Can you work these out from the drawing? Everything is in mm from the part's minimum corner. Coordinates: 2 decimals unless noted, no trailing zeros. Order: outer loops, then holes, each group sorted by start corner. A loop starts at its lowest first (then second) coordinate and runs counter-clockwise, first axis right, second up. Notation, with made-up numbers: (86.25, 73) - (90.25, 73) arc R22 cw to (90.25, 92) - close; hole circle Ø8 at (42, 71.25). An arc over 180 degrees is marked (long way). Use a Markdown table: item, result. Add a question column.
(1) I want a section at B-B (z = 1.2). List the corners of the cut face in (x, y) for me, and give its area (3 significant figures).
(2) We'd pull the mould along Y, two halves only. Please class the marked faces 1, 2 and 3: pulls with the +Y half, pulls with the -Y half, needs draft (parallel to the pull), parting line crosses it, or undercut.
(3) I want a section at C-C (y = 3). List the corners of the cut face in (x, z) for me.
(4) If I drill on L1, parallel to Z at x = 1.35, y = 5.25; L2, parallel to Z at x = 0.4, y = 4; L3, parallel to X at y = 9.5, z = 1.05, over which ranges is the centre line in solid material (lowest first)? Write a range as [from, to].
(5) I want a section at A-A (x = 1.4). List the corners of the cut face in (y, z) for me, and give its area (3 significant figures).
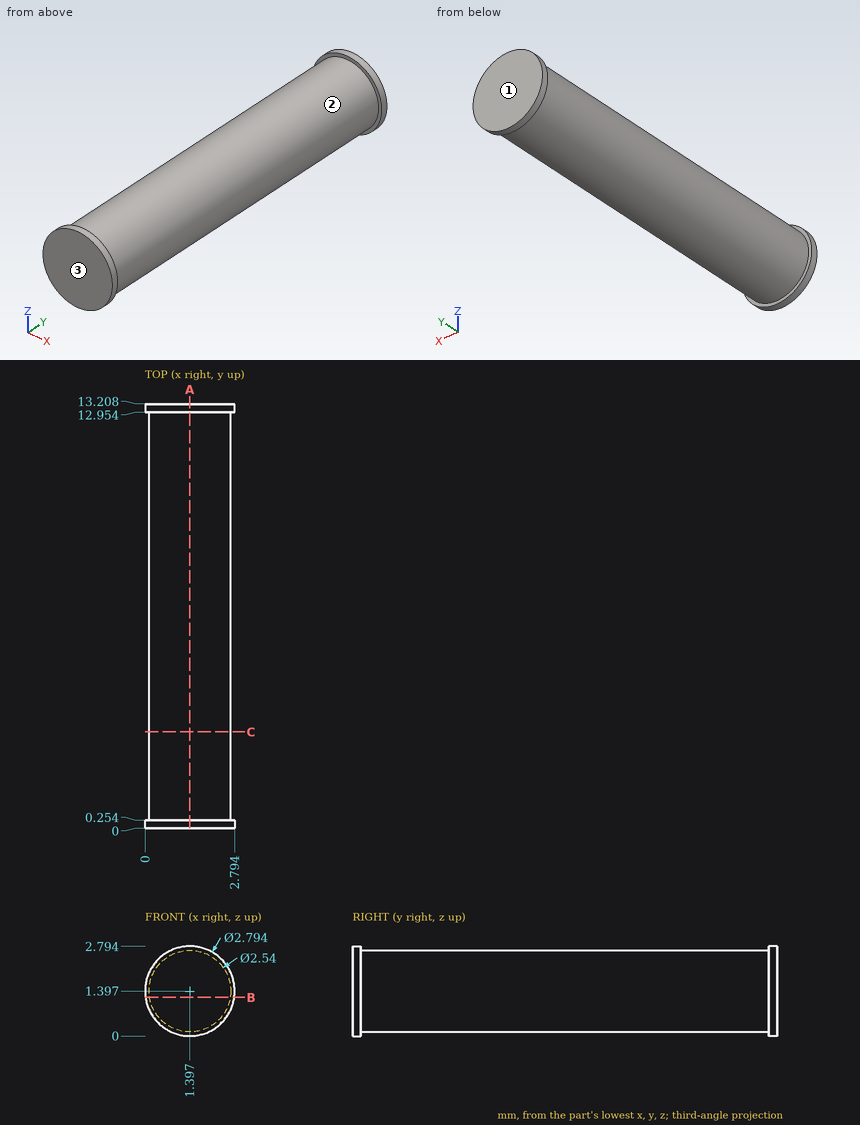
Answers follow:
| question | item | result |
|---|---|---|
| 1 | outline | (0.01, 0) - (2.78, 0) - (2.78, 0.25) - (2.65, 0.25) - (2.65, 12.95) - (2.78, 12.95) - (2.78, 13.21) - (0.01, 13.21) - (0.01, 12.95) - (0.14, 12.95) - (0.14, 0.25) - (0.01, 0.25) - close |
| 1 | area | 33.3 mm² |
| 2 | face 1 | pulls with the +Y half |
| 2 | face 2 | undercut |
| 2 | face 3 | pulls with the -Y half |
| 3 | outline | circle Ø2.54 at (1.4, 1.4) |
| 4 | L1 | z = [0.13, 2.67] |
| 4 | L2 | z = [0.61, 2.18] |
| 4 | L3 | x = [0.18, 2.62] |
| 5 | outline | (0, 0) - (0.25, 0) - (0.25, 0.13) - (12.95, 0.13) - (12.95, 0) - (13.21, 0) - (13.21, 2.79) - (12.95, 2.79) - (12.95, 2.67) - (0.25, 2.67) - (0.25, 2.79) - (0, 2.79) - close |
| 5 | area | 33.7 mm² |
